Verification items for the finished model (mm, model axes). A direction names the side the tool comes from. Coordinates: 2 decimals unless noted, no trailing zeros. Order: outer loops, then holes, each group sorted by start corner. A loop starts at its lowest first (then second) coordinate and runs counter-clockwise, first axis right, second up. Notation, with made-up numbers: M 10.25,-24.75 L 64.25,-24.75 A23 cw 64.25,4.25 Z; hole C 43,11 d1. An arc over 180 degrees is marked long. Return JSON: item names as keys, results as strings. Group by question number.
Q1. Section check B-B, the plane z = 63. Enter the section's corners in (x, y).
Q2. Mould release check, pull along X, two halves, no side actions. Record for faces 1 (the face through (94, 41, 0)), 2 (the face through (92.331, 34.587, 6.439)), 3 (the face through (25.4, 41, 36)): pulls with the +X half, pulls with the -X half, needs draft (parallel to the pull), parting line crosses it, or undercut.
Q3. Thickness scan on probe 1 along Y at (x, z) = (76.2, 7); probe 2 along X at (y, z) = (36, 9); probe 3 along X at (y, z) = (43, 8.5). Record the ranges inside material, lowest first.
Q4. Go/stop test with flat-tipped pins: pin 1 Ø8 at (y, z) = (38.5, 39) entering from +X; pin 2 Ø4 at (x, y) = (113, 13) entering from +Z; pin 3 Ø1.5 at (y, z) = (47, 27) entering from -X. Record where each tip stops, or that it passes through.
Q5. Section check D-D, the plane x = 175. Enter the section's corners in (y, z).
Q6. Section check C-C, the plane y = 29.5. Enter the section's corners in (x, z), then the cut area to 3 significant figures.
Q7. Section check A-A, the plane x = 76.2. Enter the section's corners in (y, z), then the cut area to 3 significant figures.
Q8. Access from +Z, -Z, +X, -X, +Y, -Y to the whole of each face (thin tool, end or side, straight path). Record for faces 4 (the face through (190.5, 41, 6)), 5 (the face through (109, 41, 12.7)).
from build123d import *

# Parameters (mm, degrees)
F1_DEPTH = 82.55
F2_R     = 17.4625
F3_DEPTH = 12.7
F6_DEPTH = 25.4
F7_R     = 17.4625
F8_DEPTH = 25.4


with BuildPart() as f1:
    # F0 (on Front) → F1 (new body)
    with BuildSketch(Plane.XZ):
        Polygon((0, 114.3), (0, 0), (190.5, 0), (190.5, 12.7), (25.4, 12.7), (25.4, 114.3), align=None)
    extrude(amount=-F1_DEPTH)

    # F2 (on face) → F3 (cut)
    with BuildSketch(Plane.XY.offset(12.7)):
        with Locations((76.2, 41.275)):
            Circle(F2_R)
        with Locations((152.4, 41.275)):
            Circle(F2_R)
    extrude(amount=-F3_DEPTH, mode=Mode.SUBTRACT)

    # F5 (on face) → F6 (cut)
    with BuildSketch(Plane(origin=(0, 0, 0), x_dir=(0, -1, 0), z_dir=(-1, 0, 0))):
        with BuildLine():
            ThreePointArc((-82.55, 57.15), (-41.275, 98.425), (0, 57.15))
            Line((0, 57.15), (0, 114.3))
            Line((0, 114.3), (-82.55, 114.3))
            Line((-82.55, 114.3), (-82.55, 57.15))
        make_face()
    extrude(amount=-F6_DEPTH, mode=Mode.SUBTRACT)

    # F7 (on face) → F8 (cut, through all)
    with BuildSketch(Plane.YZ.offset(25.4)):
        with Locations((41.275, 57.625926)):
            Circle(F7_R)
    extrude(amount=-F8_DEPTH, mode=Mode.SUBTRACT)


solid = f1.part
Numbers:
{
 "1": {"outline": "M 0,0.42 L 25.4,0.42 L 25.4,24.66 L 0,24.66 Z; M 0,57.89 L 25.4,57.89 L 25.4,82.13 L 0,82.13 Z"},
 "2": {"face 1": "needs draft", "face 2": "undercut", "face 3": "pulls with the +X half"},
 "3": {"probe 1": "y = 0 to 23.81, 58.74 to 82.55", "probe 2": "x = 0 to 59.55, 92.85 to 135.75, 169.05 to 190.5", "probe 3": "x = 0 to 58.82, 93.58 to 135.02, 169.78 to 190.5"},
 "4": {"pin 1": "stops at x = 25.4", "pin 2": "stops at z = 12.7", "pin 3": "stops at x = 0"},
 "5": {"outline": "M 0,0 L 82.55,0 L 82.55,12.7 L 0,12.7 Z"},
 "6": {"outline": "M 0,0 L 63.3,0 L 63.3,12.7 L 25.4,12.7 L 25.4,44.73 L 0,44.73 Z; M 0,70.52 L 25.4,70.52 L 25.4,96.71 L 0,96.71 Z; M 89.1,0 L 139.5,0 L 139.5,12.7 L 89.1,12.7 Z; M 165.3,0 L 190.5,0 L 190.5,12.7 L 165.3,12.7 Z", "area": "3,240 mm2"},
 "7": {"outline": "M 0,0 L 23.81,0 L 23.81,12.7 L 0,12.7 Z; M 58.74,0 L 82.55,0 L 82.55,12.7 L 58.74,12.7 Z", "area": "605 mm2"},
 "8": {"face 4": "+Z, -Z, +X, +Y, -Y", "face 5": "+Z, +X, +Y, -Y"}
}
